Build history of the part. All positions in model axes, mm. Face numbers are marked on the shaded views. Give positions to 0.01 mm unless a question says otherwise; leave off trailing zeros. Order: outer loops, then holes, each group sorted by start corner. A loop starts at its lowest first (then second) coordinate and runs counter-clockwise, first axis right, second up. Notation, with made-up numbers: (-39.5, -31) - (-28.5, -31) arc R9 ccw to (-28.5, -27) - close; hole circle Ø1 at (74.5, 57.5). An arc over 180 degrees is marked (long way). Write each question's results on one line, items separated by ' | '. Start each with the question number.
1) Drill centre lines: line 1 along Y through (x, z) = (0, 4.05); line 2 along Y through (x, z) = (16.5, 3.2); line 3 along X through (y, z) = (18.5, 4.5). Where is each one in solid material? Low to high. Write a range as from..to.
2) Drop flat-ended pins along their axis: pin 1 Ø3.5 at (y, z) = (-9, 3) entering from -X; pin 2 Ø4 at (x, y) = (17, -17) entering from -Z. Give the stop position or say it passes through.
3) Cut at D-D on y = 17. List the corners of the cut face in (x, z), plus the area to 3 significant figures.
4) Two-plate mould, pull along X, no slides. Class the marked faces 1, 2 and 3: +X half, -X half, draft (parallel to the pull), parting line (faces both ways), or undercut.
5) Cut at B-B on y = 0. List the corners of the cut face in (x, z), plus the area to 3 significant figures.
6) Cut at A-A on x = -17. List the corners of the cut face in (y, z), plus the area to 3 significant figures.
7) Cut at C-C on x = 17. List the corners of the cut face in (y, z), plus the area to 3 significant figures.
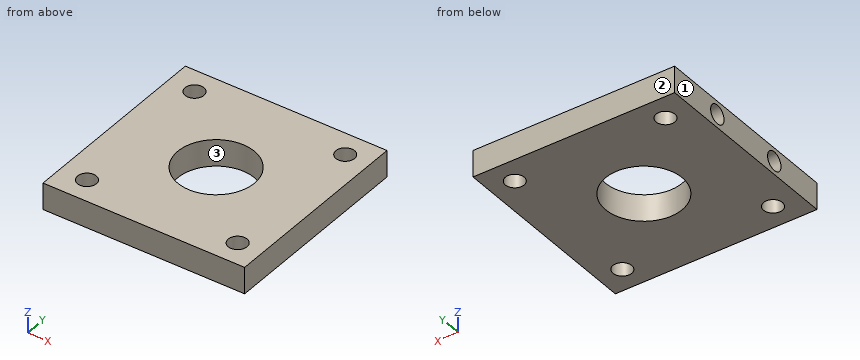
from build123d import *

# Parameters (mm, degrees)
SKETCH1_W                                     = 45.5
SKETCH1_H                                     = 45
SKETCH1_R                                     = 8.65
SKETCH1_R_2                                   = 2.12
SIX_MM_HEAD_PLATE_BOLTS_TO_34_MM_SQUARE_DEPTH = 6
MOUNTING_START                                = -23
SKETCH2_R                                     = 2.12
MOUNTING_TOE_TAPPED_FROM_BOTTOM_DEPTH         = 7


with BuildPart() as part:
    # Sketch1 → Six mm head plate bolts to 34 mm square pattern (new body)
    with BuildSketch(Plane.XY):
        with Locations((-0.25, 0)):
            Rectangle(SKETCH1_W, SKETCH1_H)
        Circle(SKETCH1_R, mode=Mode.SUBTRACT)
        with Locations((-17, -17)):
            Circle(SKETCH1_R_2, mode=Mode.SUBTRACT)
        with Locations((-17, 17)):
            Circle(SKETCH1_R_2, mode=Mode.SUBTRACT)
        with Locations((17, -17)):
            Circle(SKETCH1_R_2, mode=Mode.SUBTRACT)
        with Locations((17, 17)):
            Circle(SKETCH1_R_2, mode=Mode.SUBTRACT)
    extrude(amount=SIX_MM_HEAD_PLATE_BOLTS_TO_34_MM_SQUARE_DEPTH)

    # Sketch2 → Mounting toe tapped from bottom (cut)
    with BuildSketch(Plane(origin=(0, 0, 0), x_dir=(0, 0, -1), z_dir=(1, 0, 0)).offset(MOUNTING_START)):
        with Locations((-3, -9)):
            Circle(SKETCH2_R)
        with Locations((-3, 9)):
            Circle(SKETCH2_R)
    extrude(amount=MOUNTING_TOE_TAPPED_FROM_BOTTOM_DEPTH, mode=Mode.SUBTRACT)


solid = part.part
Results:
1) line 1: -22.5..-8.65, 8.65..22.5 | line 2: -22.5..-19.06, -14.94..14.94, 19.06..22.5 | line 3: -23..-18.5, -15.5..15.5, 18.5..22.5
2) pin 1: x = -16 | pin 2: through
3) outline: (-23, 0) - (-19.12, 0) - (-19.12, 6) - (-23, 6) - close; (-14.88, 0) - (14.88, 0) - (14.88, 6) - (-14.88, 6) - close; (19.12, 0) - (22.5, 0) - (22.5, 6) - (19.12, 6) - close | area: 222 mm^2
4) face 1: -X half | face 2: draft | face 3: undercut
5) outline: (-23, 0) - (-8.65, 0) - (-8.65, 6) - (-23, 6) - close; (8.65, 0) - (22.5, 0) - (22.5, 6) - (8.65, 6) - close | area: 169 mm^2
6) outline: (-22.5, 0) - (-19.12, 0) - (-19.12, 6) - (-22.5, 6) - close; (-14.88, 0) - (14.88, 0) - (14.88, 6) - (-14.88, 6) - close; (19.12, 0) - (22.5, 0) - (22.5, 6) - (19.12, 6) - close; hole circle Ø4.24 at (-9, 3); hole circle Ø4.24 at (9, 3) | area: 191 mm^2
7) outline: (-22.5, 0) - (-19.12, 0) - (-19.12, 6) - (-22.5, 6) - close; (-14.88, 0) - (14.88, 0) - (14.88, 6) - (-14.88, 6) - close; (19.12, 0) - (22.5, 0) - (22.5, 6) - (19.12, 6) - close | area: 219 mm^2
